Could you check a few things on this model? Use its own coordinates, in mm. Round coordinates to 2 decimals unless told otherwise and drop trailing zeros. Loops run counter-clockwise (first coordinate to the right, second up) from the corner with the lowest first, then second, coordinate; pieces in that order, holes last.
Autodesk Inventor part; units mm, degrees
ref_plane "Work Plane1" through (0, 36.5125, 304.8) normal (0, 1, 0) x (-1, 0, 0)
ref_plane "Work Plane2" through (0, 36.5125, 304.8) normal (0, 1, 0) x (-1, 0, 0)
ref_plane "YZ Plane" through (0, 0, 0) normal (1, 0, 0) x (0, 1, 0)
sketch "Sketch1" plane through (0, 0, 0) normal (0, 0, 1) x (1, 0, 0)
  circle A0 centre (0, 0) radius 36.5125
  circle A1 centre (0, 0) radius 31.3563
  dimension "d0" = 73.025
  dimension "d2" = 5.1562
extrude "Extrusion1" add sketch "Sketch1" along normal blind 304.8
sketch "Sketch2" plane through (0, 0, 304.8) normal (0, 0, 1) x (1, 0, 0)
  circle A0 centre (0, 0) radius 31.3563
  circle A1 centre (0, 0) radius 36.5125
  point P0 (0, 36.5125)
ref_plane "Work Plane1" through (0, 36.5125, 304.8) normal (0, 1, 0) x (-1, 0, 0)
sketch "Sketch5" plane through (0, 36.5125, 304.8) normal (0, 1, 0) x (-1, 0, 0)
  circle A0 centre (0, -279.4) radius 4.4901
  circle A1 centre (0, -260.35) radius 4.4901
  point P0 (0, -304.8)
  dimension "d25" = 25.4
  dimension "d26" = 19.05
hole "Hole3" at (0, 36.5125, 44.45) at (0, 36.5125, 25.4) direction (0, -1, 0) diameter 3.175 end through all
sketch "Sketch6" plane through (0, 0, 304.8) normal (0, 0, 1) x (1, 0, 0)
  circle A0 centre (0, 0) radius 31.3563
  circle A1 centre (0, 0) radius 36.5125
  point P0 (0, 36.5125)
ref_plane "Work Plane2" through (0, 36.5125, 304.8) normal (0, 1, 0) x (-1, 0, 0)
sketch "Sketch9" plane through (0, 0, 304.8) normal (0, 0, 1) x (1, 0, 0)
  circle A0 centre (0, 0) radius 31.3563
  circle A1 centre (0, 0) radius 36.5125
  line L0 (-1.27, 30.7627) -> (1.27, 30.7627)
  line L1 (1.27, 30.7627) -> (1.27, 33.3027)
  line L2 (1.27, 33.3027) -> (-1.27, 33.3027)
  line L3 (-1.27, 33.3027) -> (-1.27, 30.7627)
  line L4 (0, 33.3027) -> (0, 30.7627) construction
  line L5 (0, 31.3563) -> (0, 36.5125) construction
  dimension "d38" = 2.54
  dimension "d39" = 2.54
extrude "Extrusion3" cut sketch "Sketch9" against normal blind 25.4 contours L1 L0 L3 A0 | A0 L3 L2 L1 picked at (0.1411, 30.9596)
properties part number "2h2slv" material "PVC-Piping"
Item 1: If I drill on line 1 along Z through (x, y) = (0, 33.65); line 2 along Y through (x, z) = (0, 68.5); line 3 along X through (y, z) = (-7, 285.5), over which ranges is the centre line in solid material (lowest first)?
Results list:
line 1: z = 0 to 23.81, 26.99 to 42.86, 46.04 to 304.8
line 2: y = -36.51 to -31.36, 31.36 to 36.51
line 3: x = -35.84 to -30.56, 30.56 to 35.84
Item 2: If we section it at C-C, the plane z = 50: Please give me the cut outline in (x, y) (1 decimal), then the cut area to 3 significant figures.
Results list:
outline: circle Ø73 at (0, 0); hole circle Ø62.7 at (0, 0)
area: 1,100 mm2
Item 3: Will these pins go through, and if not, where does the flat tip stop? pin 1 (1 mm diameter, centred on y = 32.5, z = 289, fed in from +X); pin 2 (1 mm diameter, centred on y = 32.5, z = 293.5, fed in from -X); pin 3 (4 mm diameter, centred on x = 26.5, z = 84, fed in from -Y).
Results list:
pin 1: stops at x = 17.58
pin 2: stops at x = -17.58
pin 3: stops at y = -27.07
Item 4: We'd pull the mould along Y, two halves only. Please class faces 1 (the cylindrical face through (34.826, -10.967, 150.266)), 2 (the cylindrical face through (-24.883, 19.08, 150.266)), 3 (the flat face through (16.1, 27.2, 0)): released by +Y, released by -Y, zero draft, split by the parting line, or undercut.
Results list:
face 1: split by the parting line
face 2: undercut
face 3: zero draft
Item 5: If we section it at B-B, the plane x = 7: Please give me the cut outline in (y, z), then the cut area to 3 significant figures.
Results list:
outline: (-35.84, 0) - (-30.56, 0) - (-30.56, 304.8) - (-35.84, 304.8) - close; (30.56, 0) - (35.84, 0) - (35.84, 304.8) - (30.56, 304.8) - close
area: 3,210 mm2
Item 6: If we section it at A-A, the plane y = 0: Please give me the cut outline in (x, z).
Results list:
outline: (-36.51, 0) - (-31.36, 0) - (-31.36, 304.8) - (-36.51, 304.8) - close; (31.36, 0) - (36.51, 0) - (36.51, 304.8) - (31.36, 304.8) - close
